Verification items for the finished model (mm, model axes). A direction names the side the tool comes from. Coordinates: 2 decimals unless noted, no trailing zeros. Order: outer loops, then holes, each group sorted by start corner. A loop starts at its lowest first (then second) coordinate and runs counter-clockwise, first axis right, second up. Notation, with made-up numbers: (79.25, -34) -> (91.25, -34) arc R18 cw to (91.25, -6) -> close; hole circle Ø7 at (32.5, -33.5). An arc over 180 degrees is marked (long way). Write each question's results on one line, items separated by ' | '. Start each with the question number.
(1) Set-up check for faces 5 (the flat face through (-22.95, -14.98, 21.45)), 6 (the cylindrical face through (-22.008, -10.479, 21.446)), 7 (the cylindrical face through (-3.17, 24.17, 21.45)), 8 (the flat face through (22.95, 14.98, 21.45)), 9 (the cylindrical face through (34.284, -18.59, 21.446)): record each of +Z, -Z, +X, -X, +Y, -Y from which the full face is reachable in a straight line by a thin tool's end or side.
(2) Draft check along X on faces 1 (the flat face through (0, 27, 21)), 2 (the cylindrical face through (28.275, 26.861, 21.446)), 3 (the flat face through (16.163, 22.246, 21.446)), 4 (the flat face through (-6, 5, 0)). Enter one of: +X half, -X half, draft (parallel to the pull), parting line (faces both ways), or undercut.
(3) Go/stop test with flat-tipped pins: pin 1 (1.8 mm diameter, centred on y = 26, z = 30.5, fed in from -X); pin 2 (2 mm diameter, centred on x = 21, y = 26, fed in from -Z); pin 3 (3 mm diameter, centred on x = -29.5, z = 23.5, fed in from -Y); pin 4 (5 mm diameter, centred on x = -1.5, z = 37.5, fed in from -Y). Record where each tip stops, or that it passes through.
(4) Thickness scan on probe 1 along X at (y, z) = (29, 31.5); probe 2 along X at (y, z) = (35.5, 29); probe 3 along Y at (x, z) = (3, 29). Record the ranges inside material, lowest first. Write a range as [from, to].
(5) Cross-section at A-A on y = 4.5. Enter the section's corners in (x, z).
```python
from build123d import *

# Parameters (mm, degrees)
BOSS_EXTRUDE1_DEPTH = 43.5
CIRPATTERN1_COUNT   = 10
SKETCH2_R           = 7.5
CUT_EXTRUDE1_DEPTH  = 70.959609915


with BuildPart() as part:
    # Sketch1 → Boss-Extrude1 (new body)
    with BuildSketch(Plane.XY):
        with BuildLine():
            add(Edge.make_bspline(
                [(0, 30.535), (1.094025697, 33.738879921), (2.960368297, 36.423385517), (5.329249796, 38.634170065)],
                knots=[0, 0, 0, 0, 0.089409401, 0.089409401, 0.089409401, 0.089409401], degree=3))
            Line((0, 30.535), (0, 24.375))
            ThreePointArc((0, 24.375), (-4.413773565, -23.972050974), (8.681616812, 22.776526393))
            Line((8.681616812, 22.776526393), (10.875617204, 28.532563422))
            add(Edge.make_bspline(
                [(10.875617204, 28.532563422), (10.994458338, 31.915995933), (10.206644899, 35.089189117), (8.780523558, 37.998715847)],
                knots=[0, 0, 0, 0, 0.089409401, 0.089409401, 0.089409401, 0.089409401], degree=3))
            ThreePointArc((8.780523558, 37.998715847), (7.062037704, 38.355281559), (5.329249796, 38.634170065))
        make_face()
    boss_extrude1 = extrude(amount=BOSS_EXTRUDE1_DEPTH)

    # CirPattern1: Boss-Extrude1 ×10 about axis
    cirpattern1_axis = Axis((0, 0, 43.5), (0, 0, 1))
    for i in range(1, CIRPATTERN1_COUNT):
        add(boss_extrude1.rotate(cirpattern1_axis, i * 360 / CIRPATTERN1_COUNT))

    # Sketch2 → Cut-Extrude1 (cut, through all)
    with BuildSketch(Plane.XY.offset(43.5)):
        Circle(SKETCH2_R)
    extrude(amount=-CUT_EXTRUDE1_DEPTH, mode=Mode.SUBTRACT)


solid = part.part
```
Results are:
1) face 5: +Z, -Z, -X | face 6: +Z, -Z | face 7: +Z, -Z, +Y | face 8: +Z, -Z, +X | face 9: +Z, -Z, +X, -Y
2) face 1: undercut | face 2: +X half | face 3: undercut | face 4: draft
3) pin 1: stops at x = -18.48 | pin 2: stops at z = 0 | pin 3: stops at y = -27.15 | pin 4: stops at y = -37.28
4) probe 1: x = [-18.75, -7.84], [0, 10.89] | probe 2: x = [-16.15, -14.5], [2.56, 9.82] | probe 3: y = [-24.19, -6.87], [6.87, 36.09]
5) outline: (-23.96, 0) -> (-6, 0) -> (-6, 43.5) -> (-23.96, 43.5) -> close; (6, 0) -> (38.74, 0) -> (38.74, 43.5) -> (6, 43.5) -> close
